Part model, mm, in its own coordinate system. A direction names the side the tool comes from. Round coordinates to 2 decimals unless told otherwise and drop trailing zeros. Write each loop counter-clockwise with the first axis right and the second up, starting at its lowest first coordinate (ties: lowest second). Pieces come first, ordered by that corner, then holes. Notation, with made-up numbers: (-17.5, -10.75) -> (28.5, -10.75) arc R23 cw to (28.5, 18.25) -> close; hole circle Ø9 at (-32, -28.75). An arc over 180 degrees is marked (long way). Return JSON: item names as keys, results as strings. Group by question number.
(1) Saw through at B-B (y = 6). List the corners of the cut face in (x, z).
(2) Drill centre lines: L1, parallel to Z at x = 5, y = -5.25; L2, parallel to X at y = 5, z = 11; L3, parallel to Y at x = 7, z = 34.5. Where is each one in solid material? Low to high. Write a range as from..to.
(3) Tool access for faces 1 (the cylindrical face through (3.004, -2.641, 63.26)), 2 (the cylindrical face through (-3.784, -1.296, 63.26)), 3 (the flat face through (2.847, 0.986, 63.26)): list every direction of +Z, -Z, +X, -X, +Y, -Y with a clear straight run to the whole face (end or side of a thin tool).
(4) Saw through at A-A (z = 33). List the corners of the cut face in (x, y).
(5) Drop flat-ended pins along their axis: pin 1 Ø4 at (y, z) = (3, 41) entering from -X; pin 2 Ø3 at (y, z) = (4.5, 13.5) entering from +X; pin 3 Ø5 at (x, z) = (4, 30) entering from +Y. Give the stop position or say it passes through.
from build123d import *

# Parameters (mm, degrees)
SKETCH_1_R          = 8.6
EXTRUDE_1_DEPTH     = 64
SKETCH_2_OUTSIDE_W  = 32.894
SKETCH_2_OUTSIDE_H  = 32.894
CUT_EXTRUDE_1_DEPTH = 1.5


with BuildPart() as part:
    # Эскиз1 → Бобышка-Вытянуть1 (new body)
    with BuildSketch(Plane.XY):
        Circle(SKETCH_1_R)
    extrude(amount=EXTRUDE_1_DEPTH)

    # Эскиз2 outside → Вырез-Вытянуть1 (cut)
    with BuildSketch(Plane.XY.offset(64)):
        Rectangle(SKETCH_2_OUTSIDE_W, SKETCH_2_OUTSIDE_H)
        with BuildLine():
            Line((2.028187196, 3.4476741), (3.689688099, -1.544733546))
            ThreePointArc((3.689688099, -1.544733546), (2.991550535, -2.655301376), (1.971679756, -3.480298685))
            Line((1.971679756, -3.480298685), (-3.182622543, -2.422996853))
            ThreePointArc((-3.182622543, -2.422996853), (-3.790151064, -1.278575346), (-4, 0))
            Line((-4, 0), (-0.507065556, 3.967730399))
            ThreePointArc((-0.507065556, 3.967730399), (0.803783179, 3.918409448), (2.028187196, 3.4476741))
        make_face(mode=Mode.SUBTRACT)
    extrude(amount=-CUT_EXTRUDE_1_DEPTH, mode=Mode.SUBTRACT)


solid = part.part
Computed values:
{
 "1": {"outline": "(-6.16, 0) -> (6.16, 0) -> (6.16, 62.5) -> (-6.16, 62.5) -> close"},
 "2": {"L1": "0..62.5", "L2": "-7..7", "L3": "-5..5"},
 "3": {"face 1": "+Z, +X, -Y", "face 2": "+Z, -X, -Y", "face 3": "+Z, +X, +Y"},
 "4": {"outline": "circle Ø17.2 at (0, 0)"},
 "5": {"pin 1": "x = -8.54", "pin 2": "x = 8.06", "pin 3": "y = 8.47"}
}
